Input: dimensioned drawing with shaded views. Units: mm. Origin: part minimum x, y, z. Coordinates: 2 decimals unless noted, no trailing zeros. Order: outer loops, then holes, each group sorted by start corner. A loop starts at its lowest first (then second) coordinate and runs counter-clockwise, first axis right, second up. Notation, with made-up numbers: (84, 52) -> (107, 52) arc R17 ccw to (107, 66) -> close; hole circle Ø3 at (39, -38). An arc over 180 degrees is marked (long way). Answer as CSV lines item,"result".
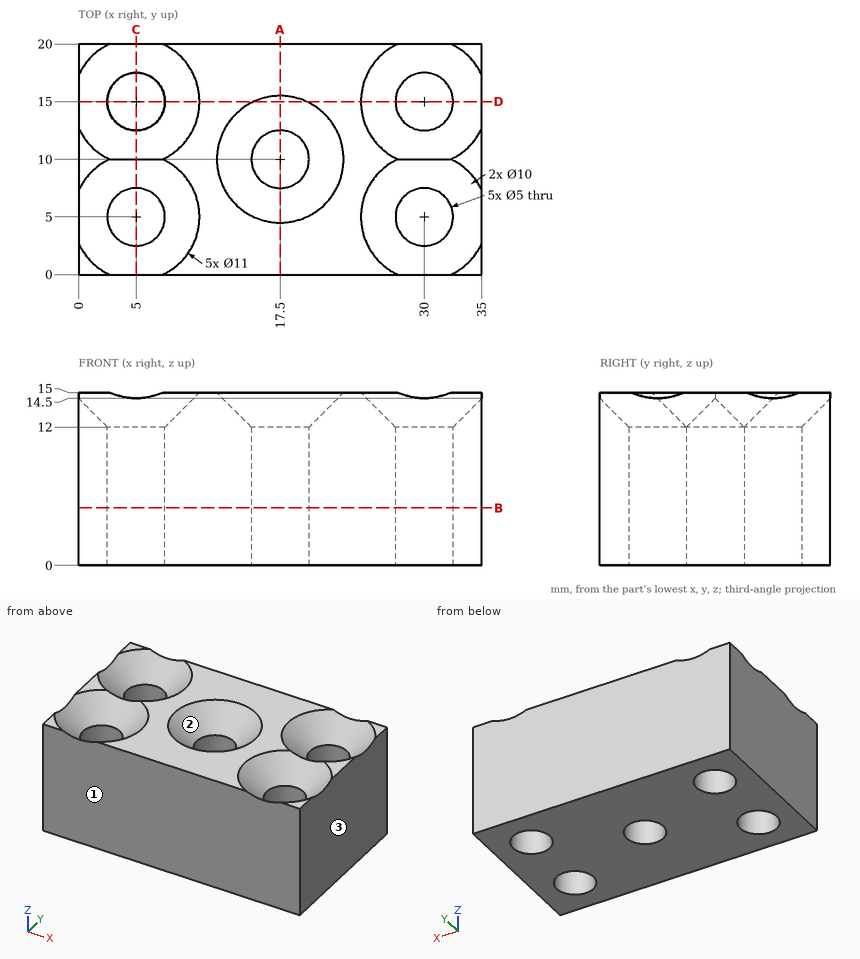
1. Ray query, line 1 along Y through (x, z) = (30, 3.25); line 2 along X through (y, z) = (4.25, 3.25); line 3 along X through (y, z) = (6.5, 8.75). Return the intervals inside material, ascending.
Findings:
line 1,"y = 0 to 2.5, 7.5 to 12.5, 17.5 to 20"
line 2,"x = 0 to 2.62, 7.38 to 27.62, 32.38 to 35"
line 3,"x = 0 to 3, 7 to 28, 32 to 35"
2. Cut plane D-D (y = 15). State how many separate pieces and enclosed holes the cut face has, plus the area to 3 significant figures.
Findings:
separate pieces,"3"
enclosed holes,"0"
area,"356 mm2"
3. Cut plane A-A (x = 17.5). Return the cut outline in (y, z).
Findings:
outline,"(0, 0) -> (7.5, 0) -> (7.5, 12) -> (4.5, 15) -> (0, 15) -> close; (12.5, 0) -> (20, 0) -> (20, 15) -> (15.5, 15) -> (12.5, 12) -> close"
4. Mould query, pull axis X, two halves, no side actions, for the marked faces 1, 2 and 3. Classes: released by +X, released by -X, zero draft, split by the parting line, or undercut.
Findings:
face 1,"zero draft"
face 2,"undercut"
face 3,"released by +X"
5. Contact query for flat-ended pins moving along their axis: pin 1 (2 mm diameter, centred on x = 12.5, y = 9.5, fed in from -Z); pin 2 (3 mm diameter, centred on x = 17.5, y = 10, fed in from +Z). Output: stop coordinate, or through.
Findings:
pin 1,"stops at z = 0"
pin 2,"passes through"
6. Cut plane B-B (z = 5). Return the cut outline in (x, y), plus the area to 3 significant figures.
Findings:
outline,"(0, 0) -> (35, 0) -> (35, 20) -> (0, 20) -> close; hole circle Ø5 at (5, 5); hole circle Ø5 at (5, 15); hole circle Ø5 at (17.5, 10); hole circle Ø5 at (30, 5); hole circle Ø5 at (30, 15)"
area,"602 mm2"
7. Cut plane C-C (x = 5). Return the cut outline in (y, z).
Findings:
outline,"(0, 0) -> (2.5, 0) -> (2.5, 12) -> (0, 14.5) -> close; (7.5, 0) -> (12.5, 0) -> (12.5, 12) -> (10, 14.5) -> (7.5, 12) -> close; (17.5, 0) -> (20, 0) -> (20, 14.5) -> (17.5, 12) -> close"
